The listing builds one solid part. Answer for the finished solid, in the listing's coordinates (mm). A direction names the side the tool comes from. Coordinates: 2 decimals unless noted, no trailing zeros. Loops run counter-clockwise (first coordinate to the right, second up) from the corner with the lowest first, then second, coordinate; pieces in that order, holes last. Notation, with made-up numbers: (78.25, 8) - (107.25, 8) arc R20 cw to (107.25, 47) - close; hole circle Ø6 at (88.25, 69.25). An arc over 180 degrees is marked (long way). One line per question, with ' | ' between items.
from build123d import *

# Parameters (mm, degrees)
SKETCH006_R                = 5
PAD005_DEPTH               = 9
PAD006_DEPTH               = 4
SKETCH009_R                = 2.25
PAD008_DEPTH               = 13
POCKET_DEPTH               = 13
POCKET_MIRRORED004_2_DEPTH = 13


with BuildPart() as part:
    # Sketch006 (on Face30 of Binder) → Pad005 (new body)
    with BuildSketch(Plane(origin=(0, 0, 0), x_dir=(1, 0, 0), z_dir=(0, 0, -1))):
        Polygon((-24.5, -24.5), (24.5, -24.5), (24.5, -6), (13.5, -6), (13.5, 6), (24.5, 6), (24.5, 24.5), (-24.5, 24.5), align=None)
        with Locations((-7, 17.5)):
            Circle(SKETCH006_R, mode=Mode.SUBTRACT)
        with Locations((-7, -17.5)):
            Circle(SKETCH006_R, mode=Mode.SUBTRACT)
    extrude(amount=PAD005_DEPTH)

    # Sketch007 (on Face11 of Pad005) → Pad006 (join)
    with BuildSketch(Plane.XY):
        Polygon((-20.25, 20.25), (-20.25, -20.25), (20.25, -20.25), (20.25, -6), (24.5, -6), (24.5, -24.5), (-24.5, -24.5), (-24.5, 24.5), (24.5, 24.5), (24.5, 6), (20.25, 6), (20.25, 20.25), align=None)
    extrude(amount=PAD006_DEPTH)

    # Sketch009 (on Face7 of Pad006) → Pad008 (join)
    with BuildSketch(Plane.XY.offset(4)):
        with BuildLine():
            ThreePointArc((-5, 34), (-8.18198, 32.681981), (-9.5, 29.5))
            Line((-9.5, 29.5), (-9.5, 24.5))
            Line((-9.5, 24.5), (9.5, 24.5))
            Line((9.5, 29.5), (9.5, 24.5))
            ThreePointArc((9.5, 29.5), (8.181981, 32.681981), (5, 34))
            Line((5, 34), (-5, 34))
        make_face()
        with Locations((5, 29.5)):
            Circle(SKETCH009_R, mode=Mode.SUBTRACT)
        with Locations((-5, 29.5)):
            Circle(SKETCH009_R, mode=Mode.SUBTRACT)
    pad008 = extrude(amount=-PAD008_DEPTH)

    # Mirrored001: Pad008 across Sketch009 H_Axis
    add(pad008.mirror(Plane(origin=(0, 0, 4), x_dir=(0, 0, 1), z_dir=(0, 1, 0))))

    # Sketch018 (on Face36 of Mirrored001) → Pocket (cut)
    with BuildSketch(Plane.XY.offset(4)):
        with BuildLine():
            ThreePointArc((-24.5, -21.5), (-23.62132, -23.62132), (-21.5, -24.5))
            Line((-21.5, -24.5), (-24.5, -24.5))
            Line((-24.5, -24.5), (-24.5, -21.5))
        make_face()
    pocket = extrude(amount=-POCKET_DEPTH, mode=Mode.SUBTRACT)

    # Sketch018 Mirrored004 2 → Pocket Mirrored004 2 (cut)
    with BuildSketch(Plane(origin=(0, 0, 4), x_dir=(1, 0, 0), z_dir=(0, 0, -1))):
        with BuildLine():
            ThreePointArc((-24.5, -21.5), (-23.62132, -23.62132), (-21.5, -24.5))
            Line((-21.5, -24.5), (-24.5, -24.5))
            Line((-24.5, -24.5), (-24.5, -21.5))
        make_face()
    pocket_mirrored004_2 = extrude(amount=POCKET_MIRRORED004_2_DEPTH, mode=Mode.SUBTRACT)

    # Mirrored005: Pocket, Pocket Mirrored004 2 across Sketch018 V_Axis
    add(pocket.mirror(Plane(origin=(0, 0, 4), x_dir=(0, 0, 1), z_dir=(1, 0, 0))), mode=Mode.SUBTRACT)
    add(pocket_mirrored004_2.mirror(Plane(origin=(0, 0, 4), x_dir=(0, 0, 1), z_dir=(1, 0, 0))), mode=Mode.SUBTRACT)


solid = part.part
Item 1: The mould has two halves that part along Y. Classify faces 1 (the face through (23.64, 23.6, -2.41)), 2 (the face through (-8.147, -32.717, -2.409)), 3 (the face through (-4.693, -13.064, -4.437)): pulls with the +Y half, pulls with the -Y half, needs draft (parallel to the pull), parting line crosses it, or undercut.
Taken from the geometry:
face 1: pulls with the +Y half | face 2: pulls with the -Y half | face 3: undercut
Item 2: Which of the six approach directions +Z, -Z, +X, -X, +Y, -Y give full straight-line access (tool end or side, diameter ignored) to faces 4 (the face through (13.5, 0, -4)), 5 (the face through (-7, 21, 0)), 6 (the face through (16, -24.5, -3)), 7 (the face through (-9.5, 27, -2)), 8 (the face through (0, 0, 0))?
Taken from the geometry:
face 4: +Z, -Z, +X | face 5: -Z | face 6: +Z, -Z, +X, -Y | face 7: +Z, -Z, -X, +Y | face 8: +Z
Item 3: Find section B-B, the plane z = -7.75. State how many separate pieces and enclosed holes the cut face has, plus the area to 3 significant figures.
Taken from the geometry:
separate pieces: 1 | enclosed holes: 6 | area: 2,380 mm2
Item 4: Find section C-C, the plane x = 19.5. Write down the section's boundary in (y, z).
Taken from the geometry:
outline: (-24.5, -9) - (-6, -9) - (-6, 0) - (-20.25, 0) - (-20.25, 4) - (-24.5, 4) - close; (6, -9) - (24.5, -9) - (24.5, 4) - (20.25, 4) - (20.25, 0) - (6, 0) - close
Item 5: Find the intervals of material crossed by line 1 (Y direction, x = 5, z = -4.5); line 2 (X direction, y = -29.5, z = 0.5); line 3 (Y direction, x = -7, z = -3.75), in increasing order. Write a range as [from, to].
Taken from the geometry:
line 1: y = [-34, -31.75], [-27.25, 27.25], [31.75, 34] | line 2: x = [-9.5, -7.25], [-2.75, 2.75], [7.25, 9.5] | line 3: y = [-33.53, -30.53], [-28.47, -22.5], [-12.5, 12.5], [22.5, 28.47], [30.53, 33.53]
Item 6: Find section A-A, the plane y = -17.5. Write down the section's boundary in (x, z), plus the area to 3 significant figures.
Taken from the geometry:
outline: (-24.5, -9) - (-12, -9) - (-12, 0) - (-20.25, 0) - (-20.25, 4) - (-24.5, 4) - close; (-2, -9) - (24.5, -9) - (24.5, 4) - (20.25, 4) - (20.25, 0) - (-2, 0) - close | area: 385 mm2
Item 7: Find section D-D, the plane y = 8.5. Write down the section's boundary in (x, z), plus the area to 3 significant figures.
Taken from the geometry:
outline: (-24.5, -9) - (24.5, -9) - (24.5, 4) - (20.25, 4) - (20.25, 0) - (-20.25, 0) - (-20.25, 4) - (-24.5, 4) - close | area: 475 mm2
Item 8: Each of these flat-tipped pins is pushed along its axis until it touches: pin 1 Ø2 at (y, z) = (0, 1.5) entering from +X; pin 2 Ø2.5 at (x, y) = (-7.5, -21) entering from -Z; pin 3 Ø2 at (x, z) = (11, -0.5) entering from +Y. Where does it stop, or does it pass through?
Taken from the geometry:
pin 1: stops at x = -20.25 | pin 2: stops at z = 0 | pin 3: stops at y = 24.5
